The listing builds one solid part. Answer for the finished solid, in the listing's coordinates (mm). A direction names the side the tool comes from. Round coordinates to 2 decimals unless told otherwise and drop trailing zeros. Order: outer loops, then holes, each group sorted by start corner. A loop starts at its lowest first (then second) coordinate and runs counter-clockwise, first axis right, second up. Notation, with made-up numbers: (12, 39.25) -> (45, 39.25) arc R21 ccw to (45, 69.25) -> close; hole circle Ø9 at (64.5, 86.5). An arc over 180 degrees is marked (long way). Answer in a Markdown table with one row per item. Add a question column.
```python
from build123d import *

# Parameters (mm, degrees)
SKETCH_3_R          = 3.1
SKETCH_3_R_2        = 1.6
EXTRUDE_1_DEPTH     = 22
CUT_EXTRUDE_1_REACH = 32.691
CUT_EXTRUDE_2_DEPTH = 1.7
CUT_EXTRUDE_3_REACH = 33.141
SKETCH_6_R          = 0.8
SKETCH_7_R          = 1.4
CUT_EXTRUDE_4_DEPTH = 0.5


with BuildPart() as part:
    # 草图3 → 凸台-拉伸1 (new body)
    # profile 1 of 3: a face of its own
    with BuildSketch(Plane.XY):
        with Locations((18.05, -11.455)):
            Circle(SKETCH_3_R)
        with Locations((18.05, -11.455)):
            Circle(SKETCH_3_R_2, mode=Mode.SUBTRACT)
    # profile 2 of 3: a face of its own
    with BuildSketch(Plane.XY):
        with BuildLine():
            Line((18.05, -8.355), (-18.05, -8.355))
            ThreePointArc((-18.05, -8.355), (-15.913472443, -9.208836604), (-14.953877425, -11.3))
            Line((-14.953877425, -11.3), (14.953877425, -11.3))
            ThreePointArc((14.953877425, -11.3), (15.913472443, -9.208836604), (18.05, -8.355))
        make_face()
    # profile 3 of 3: a face of its own
    with BuildSketch(Plane.XY):
        with Locations((-18.05, -11.455)):
            Circle(SKETCH_3_R)
        with Locations((-18.05, -11.455)):
            Circle(SKETCH_3_R_2, mode=Mode.SUBTRACT)
    extrude(amount=-EXTRUDE_1_DEPTH)

    # 草图4 → 切除-拉伸1 (cut, up to next)
    with BuildSketch(Plane.XZ.offset(11.3), mode=Mode.PRIVATE) as cut_extrude_1_sk1:
        with BuildLine():
            Line((-0.25, -14.7), (0.25, -14.7))
            ThreePointArc((0.25, -14.7), (1.25, -15.7), (0.25, -16.7))
            Line((0.25, -16.7), (-0.25, -16.7))
            ThreePointArc((-0.25, -16.7), (-1.25, -15.7), (-0.25, -14.7))
        make_face()
    cut_extrude_1_tool1 = extrude(cut_extrude_1_sk1.sketch, amount=-CUT_EXTRUDE_1_REACH, mode=Mode.PRIVATE) & part.part
    add(cut_extrude_1_tool1.solids().sort_by_distance((0, -11.3, -15.7))[0], mode=Mode.SUBTRACT)

    # 草图5 → 切除-拉伸2 (cut)
    with BuildSketch(Plane(origin=(0, -8.355, 0), x_dir=(1, 0, 0), z_dir=(0, 1, 0))):
        Polygon((2.059401077, 15.7), (0.904700538, 17.7), (-1.404700538, 17.7), (-2.559401077, 15.7), (-1.404700538, 13.7), (0.904700538, 13.7), align=None)
        Polygon((2.559401077, 15.7), (1.404700538, 17.7), (-0.904700538, 17.7), (-2.059401077, 15.7), (-0.904700538, 13.7), (1.404700538, 13.7), align=None)
    extrude(amount=-CUT_EXTRUDE_2_DEPTH, mode=Mode.SUBTRACT)

    # 草图6 → 切除-拉伸3 (cut, up to next)
    with BuildSketch(Plane(origin=(0, -8.355, 0), x_dir=(1, 0, 0), z_dir=(0, 1, 0)), mode=Mode.PRIVATE) as cut_extrude_3_sk1:
        with Locations(Location((-5, 3, 0), (0, 0, 180))):
            Circle(SKETCH_6_R)
    cut_extrude_3_tool1 = extrude(cut_extrude_3_sk1.sketch, amount=-CUT_EXTRUDE_3_REACH, mode=Mode.PRIVATE) & part.part
    # 草图6 → 切除-拉伸3 (cut, up to next)
    with BuildSketch(Plane(origin=(0, -8.355, 0), x_dir=(1, 0, 0), z_dir=(0, 1, 0)), mode=Mode.PRIVATE) as cut_extrude_3_sk2:
        with Locations(Location((5, 3, 0), (0, 0, 180))):
            Circle(SKETCH_6_R)
    cut_extrude_3_tool2 = extrude(cut_extrude_3_sk2.sketch, amount=-CUT_EXTRUDE_3_REACH, mode=Mode.PRIVATE) & part.part
    add(cut_extrude_3_tool1.solids().sort_by_distance((-5, -8.355, -3))[0], mode=Mode.SUBTRACT)
    add(cut_extrude_3_tool2.solids().sort_by_distance((5, -8.355, -3))[0], mode=Mode.SUBTRACT)

    # 草图7 → 切除-拉伸4 (cut)
    with BuildSketch(Plane.XZ.offset(11.3)):
        with Locations(Location((5, -3, 0), (0, 0, 270))):
            Circle(SKETCH_7_R)
        with Locations(Location((-5, -3, 0), (0, 0, 270))):
            Circle(SKETCH_7_R)
    extrude(amount=-CUT_EXTRUDE_4_DEPTH, mode=Mode.SUBTRACT)


solid = part.part
```
Item 1: The part is cut by section A-A, the plane x = 5. Give the vertices of the cut face in (y, z) (3 decimals).
Item 2: Flat-ended cylindrical pins translate along their axes: P1, Ø10, axis at x = -5, z = -6.5, coming from the -Y side; P2, Ø1.3, axis at x = -5, z = -3, coming from the -Y side; P3, Ø0.8, axis at x = 5.5, z = -3.5, coming from the -Y side; P4, Ø2, axis at y = -13.5, z = -13, coming from the +X side. Find the tip coordinate at first contact, or state that the pin passes through.
Item 3: Find the intervals of material crossed by probe 1 along X at (y, z) = (-11.5, -3.25); probe 2 along X at (y, z) = (-10.75, -3.25); probe 3 along X at (y, z) = (-12.25, -20.25), in increasing order. Write a range as [from, to].
Item 4: The part is cut by section B-B, the plane z = -3. Give the vertices of the cut face in (x, y) (3 decimals), and give its area (3 significant figures).
Item 5: A tool of negligible diameter and unlimited length cuts with its end or side. For faces 1 (the face through (1.25, -10.69, -15.68)), 2 (the face through (6.18, -11.05, -3.75)), 3 (the face through (0, -10.055, -14)), 4 (the face through (0, -8.355, -11)), from which of +Z, -Z, +X, -X, +Y, -Y can it reach the whole face along a straight path? Write none if from no direction.
Item 6: The part is cut by section C-C, the plane y = -12. Give the vertices of the cut face in (x, z).
Item 7: The part is cut by section D-D, the plane z = -10.75. Give the vertices of the cut face in (x, y) (3 decimals).
Item 8: For a pull along X with two mould halves and no side action, classify faces 5 (the face through (0, -10, 0)), 6 (the face through (-1.974, -9.193, -16.714)), 7 (the face through (0, -11.3, -11)) as released by +X, released by -X, zero draft, split by the parting line, or undercut.
Resolved:
| question | item | result |
|---|---|---|
| 1 | outline | (-11.3, -22) -> (-8.355, -22) -> (-8.355, -3.8) -> (-10.8, -3.8) -> (-10.8, -4.4) -> (-11.3, -4.4) -> close; (-11.3, -1.6) -> (-10.8, -1.6) -> (-10.8, -2.2) -> (-8.355, -2.2) -> (-8.355, 0) -> (-11.3, 0) -> close |
| 2 | P1 | y = -11.3 |
| 2 | P2 | through |
| 2 | P3 | y = -10.8 |
| 2 | P4 | x = 20.97 |
| 3 | probe 1 | [-21.15, -19.65], [-16.45, -14.95], [14.95, 16.45], [19.65, 21.15] |
| 3 | probe 2 | [-21.07, -19.49], [-16.61, -5.76], [-4.24, 4.24], [5.76, 16.61], [19.49, 21.07] |
| 3 | probe 3 | [-21.05, -19.44], [-16.66, -15.05], [15.05, 16.66], [19.44, 21.05] |
| 4 | outline | (-18.05, -8.355) arc R3.1 ccw (long way) to (-14.954, -11.3) -> (-6.4, -11.3) -> (-6.4, -10.8) -> (-5.8, -10.8) -> (-5.8, -8.355) -> close; (-4.2, -10.8) -> (-3.6, -10.8) -> (-3.6, -11.3) -> (3.6, -11.3) -> (3.6, -10.8) -> (4.2, -10.8) -> (4.2, -8.355) -> (-4.2, -8.355) -> close; (5.8, -10.8) -> (6.4, -10.8) -> (6.4, -11.3) -> (14.954, -11.3) arc R3.1 ccw (long way) to (18.05, -8.355) -> (5.8, -8.355) -> close; hole circle Ø3.2 at (-18.05, -11.455); hole circle Ø3.2 at (18.05, -11.455) |
| 4 | area | 126 mm2 |
| 5 | face 1 | +Y, -Y |
| 5 | face 2 | -Y |
| 5 | face 3 | +Y |
| 5 | face 4 | +Z, -Z, +X, -X, +Y |
| 6 | outline | (-21.1, -22) -> (-19.55, -22) -> (-19.55, 0) -> (-21.1, 0) -> close; (-16.55, -22) -> (-15, -22) -> (-15, 0) -> (-16.55, 0) -> close; (15, -22) -> (16.55, -22) -> (16.55, 0) -> (15, 0) -> close; (19.55, -22) -> (21.1, -22) -> (21.1, 0) -> (19.55, 0) -> close |
| 7 | outline | (-18.05, -8.355) arc R3.1 ccw (long way) to (-14.954, -11.3) -> (14.954, -11.3) arc R3.1 ccw (long way) to (18.05, -8.355) -> close; hole circle Ø3.2 at (-18.05, -11.455); hole circle Ø3.2 at (18.05, -11.455) |
| 8 | face 5 | zero draft |
| 8 | face 6 | undercut |
| 8 | face 7 | undercut |
